```python
from build123d import *

# Parameters (mm, degrees)
SKETCH_1_W          = 20
SKETCH_1_H          = 3.3
EXTRUDE_1_DEPTH     = 25
SKETCH_2_R          = 1.5
CUT_EXTRUDE_1_DEPTH = 13.5
SKETCH_3_R          = 1.5
CUT_EXTRUDE_2_DEPTH = 13.5
FILLET_6_R          = 10
FILLET_7_R          = 1.5
CHAMFER_1_SIZE      = 5
FILLET_8_R          = 10


with BuildPart() as part:
    # Эскиз1 → Бобышка-Вытянуть1 (new body)
    with BuildSketch(Plane(origin=(0, 0, 0), x_dir=(1, 0, 0), z_dir=(0, 1, 0))):
        Polygon((-12.5, -25), (0, -25), (0, -50), (12.5, -50), (12.5, 50), (0, 50), (0, 25), (-12.5, 25), align=None)
        with Locations((0, 16.75)):
            Rectangle(SKETCH_1_W, SKETCH_1_H, mode=Mode.SUBTRACT)
        with Locations((0, -16.75)):
            Rectangle(SKETCH_1_W, SKETCH_1_H, mode=Mode.SUBTRACT)
    extrude(amount=EXTRUDE_1_DEPTH)

    # Эскиз2 → Вырез-Вытянуть1 (cut, through all)
    with BuildSketch(Plane.ZY):
        with Locations((-45, 6.5)):
            Circle(SKETCH_2_R)
        with Locations((-45, 18.5)):
            Circle(SKETCH_2_R)
    extrude(amount=-CUT_EXTRUDE_1_DEPTH, mode=Mode.SUBTRACT)

    # Эскиз3 → Вырез-Вытянуть2 (cut, through all)
    with BuildSketch(Plane.ZY):
        with Locations((45, 6.5)):
            Circle(SKETCH_3_R)
        with Locations((45, 18.5)):
            Circle(SKETCH_3_R)
    extrude(amount=-CUT_EXTRUDE_2_DEPTH, mode=Mode.SUBTRACT)

    # Скругление6
    fillet_6_edges = [part.edges().sort_by_distance(p)[0] for p in [
        (-12.5, 12.5, 25),
        (-12.5, 12.5, -25),
    ]]
    fillet(fillet_6_edges, radius=FILLET_6_R)

    # Скругление7
    fillet_7_edges = [part.edges().sort_by_distance(p)[0] for p in [
        (-10, 12.5, -18.4),
        (-10, 12.5, -15.1),
        (10, 12.5, -15.1),
        (10, 12.5, -18.4),
        (-10, 12.5, 15.1),
        (-10, 12.5, 18.4),
        (10, 12.5, 18.4),
        (10, 12.5, 15.1),
    ]]
    fillet(fillet_7_edges, radius=FILLET_7_R)

    # Фаска1
    chamfer_1_edges = [part.edges().sort_by_distance(p)[0] for p in [
        (6.25, 25, 50),
        (6.25, 25, -50),
    ]]
    chamfer(chamfer_1_edges, length=CHAMFER_1_SIZE)

    # Скругление8
    fillet_8_edges = [part.edges().sort_by_distance(p)[0] for p in [
        (0, 12.5, 25),
        (0, 12.5, -25),
    ]]
    fillet(fillet_8_edges, radius=FILLET_8_R)


solid = part.part
```
Work out the finished part from the listing and answer in its coordinate system (mm). A direction names the side the tool comes from. Give positions to 0.01 mm unless a question says otherwise; leave off trailing zeros. Order: outer loops, then holes, each group sorted by start corner. A loop starts at its lowest first (then second) coordinate and runs counter-clockwise, first axis right, second up. Notation, with made-up numbers: (-39.5, 39) - (-35.5, 39) arc R18 ccw to (-35.5, 63) - close; hole circle Ø7 at (-18.5, -31.5). An arc over 180 degrees is marked (long way). One line per item, written item: value. Start each with the question number.
1. Section B-B, the plane x = 11 is taken. Write down the section's boundary in (y, z), then the cut area to 3 significant figures.
2. Section C-C, the plane y = 6.5 is taken. Count the separate pieces of the cut face and the enclosed holes in it, then the cut area to 3 significant figures.
3. Which of the six approach directions +Z, -Z, +X, -X, +Y, -Y give full straight-line access (tool end or side, diameter ignored) to faces 4 (the face through (0, 12, -15.1)), 5 (the face through (3, 0, -1)), 6 (the face through (0, 12, 42))?
4. Section A-A, the plane x = 7 is taken. Write down the section's boundary in (y, z).
5. Consider line 1 (Y direction, x = 4.5, z = 45); line 2 (Z direction, x = 3.5, y = 14.5); line 3 (X direction, y = 1.5, z = 45.5). Determine where each line is inside the solid, lowest interval first.
6. For a pull along X with two mould halves and no side action, classify faces 1 (the face through (0, 12, -42)), 2 (the face through (12.5, 12, 1)), 3 (the face through (0, 12, 18.4)) as released by +X, released by -X, zero draft, split by the parting line, or undercut.
7. Each of these flat-tipped pins is pushed along its axis until it touches: pin 1 Ø5 at (y, z) = (9.5, -33) entering from -X; pin 2 Ø13 at (y, z) = (16.5, 45) entering from -X; pin 3 Ø2.5 at (y, z) = (18.5, 45) entering from -X; pin 4 Ø2 at (y, z) = (12.5, -21.5) entering from -X. Where does it stop, or does it pass through?
Filled sheet:
1. outline: (0, -50) - (20, -50) - (25, -45) - (25, 45) - (20, 50) - (0, 50) - close; hole circle Ø3 at (6.5, -45); hole circle Ø3 at (6.5, 45); hole circle Ø3 at (18.5, -45); hole circle Ø3 at (18.5, 45)
1. area: 2,450 mm²
2. separate pieces: 3
2. enclosed holes: 2
2. area: 1,650 mm²
3. face 4: +Y, -Y
3. face 5: +Z, -Z, +X, -X, -Y
3. face 6: +Z, -X, +Y, -Y
4. outline: (0, -50) - (20, -50) - (25, -45) - (25, -18.4) - (0, -18.4) - close; (0, -15.1) - (25, -15.1) - (25, 15.1) - (0, 15.1) - close; (0, 18.4) - (25, 18.4) - (25, 45) - (20, 50) - (0, 50) - close; hole circle Ø3 at (6.5, -45); hole circle Ø3 at (6.5, 45); hole circle Ø3 at (18.5, -45); hole circle Ø3 at (18.5, 45)
5. line 1: 0 to 5, 8 to 17, 20 to 25
5. line 2: -50 to -18.4, -15.1 to 15.1, 18.4 to 50
5. line 3: 0 to 12.5
6. face 1: released by -X
6. face 2: released by +X
6. face 3: undercut
7. pin 1: x = -0.47
7. pin 2: x = 0
7. pin 3: through
7. pin 4: x = -10.85
